Model file for the job. Use its own axes, mm. A direction names the side the tool comes from. Coordinates: 2 decimals unless noted, no trailing zeros. Order: outer loops, then holes, each group sorted by start corner. A loop starts at its lowest first (then second) coordinate and runs counter-clockwise, first axis right, second up. Notation, with made-up numbers: (-33.5, -25.75) -> (-0.5, -25.75) arc R32 ccw to (-0.5, 11.25) -> close; hole circle Ø11 at (4, -0.5). An arc over 180 degrees is marked (long way). Return JSON: item names as keys, results as strings. Group by question number.
1) Cut at B-B (x = -70). Write the cut outline in (y, z), and give its area (3 significant figures).
2) Cut at C-C (z = 0). State how many separate pieces and enclosed holes the cut face has, and give its area (3 significant figures).
3) Pull direction Z, two halves, no side cores. Call faces 1 (the flat face through (-20.5, -38, 0)), 2 (the cylindrical face through (59, 13, 0)): +Z half, -Z half, draft (parallel to the pull), parting line (faces both ways), or undercut.
4) Flat gauge pins, fed straight in: pin 1 (16 mm diameter, centred on y = 52.5, z = 3, fed in from +X); pin 2 (12 mm diameter, centred on y = -60.5, z = 2, fed in from -X); pin 3 (12 mm diameter, centred on x = -80, z = -4, fed in from +Y). Where does each tip first touch, or does it go through?
5) Which spindle directions (+Z, -Z, +X, -X, +Y, -Y) get a long thin tool onto all of the face, cutting with end or side? Do faces 3 (the flat face through (61, -20, 9)), 4 (the flat face through (-80, 20, 9)), 5 (the flat face through (25, 75, 0)), 6 (the flat face through (85.5, 0, 0)), 7 (the flat face through (-20.5, 53, 0)). Say none if no direction does.
6) Probe line 1 (X direction, y = 14.5, z = 0); line 2 (X direction, y = -15.75, z = 0); line 3 (Z direction, x = 70, y = -10.25). List the from-to ranges inside material, lowest first.
7) Cut at A-A (y = -47). Write the cut outline in (x, z).
from build123d import *

# Parameters (mm, degrees)
F0_W      = 60
F0_H      = 40
F1_DEPTH  = 90
F2_W      = 41
F2_H      = 40
F3_DEPTH  = 80
F4_W      = 41
F4_H      = 40
F5_DEPTH  = 80
F6_W      = 75
F6_H      = 40
F6_R      = 11
F7_DEPTH  = 20
F8_W      = 31
F8_H      = 12
F9_DEPTH  = 40
F10_R     = 20
F11_R     = 5
F12_R     = 5
F13_W     = 5
F13_H     = 30
F14_DEPTH = 80


with BuildPart() as f1:
    # F0 (on Front) → F1 (new body, symmetric)
    with BuildSketch(Plane.XZ):
        Rectangle(F0_W, F0_H)
    extrude(amount=F1_DEPTH, both=True)

    # F2 (on face) → F3 (cut)
    with BuildSketch(Plane.XZ.offset(90)):
        Rectangle(F2_W, F2_H)
    extrude(amount=-F3_DEPTH, mode=Mode.SUBTRACT)

    # F4 (on face) → F5 (cut)
    with BuildSketch(Plane(origin=(0, 90, 0), x_dir=(-1, 0, 0), z_dir=(0, 1, 0))):
        Rectangle(F4_W, F4_H)
    extrude(amount=-F5_DEPTH, mode=Mode.SUBTRACT)

    # F6 (on Front) → F7 (join, symmetric)
    with BuildSketch(Plane.XZ):
        with Locations((58, 0)):
            Rectangle(F6_W, F6_H)
        with Locations((70, 0)):
            Circle(F6_R, mode=Mode.SUBTRACT)
        with Locations((-58, 0)):
            Rectangle(F6_W, F6_H)
        with Locations((-70, 0)):
            Circle(F6_R, mode=Mode.SUBTRACT)
    extrude(amount=F7_DEPTH, both=True)

    # F8 (on face) → F9 (cut)
    with BuildSketch(Plane.XY.offset(20)):
        with Locations((70, 0)):
            Rectangle(F8_W, F8_H)
        with Locations((-70, 0)):
            Rectangle(F8_W, F8_H)
    extrude(amount=-F9_DEPTH, mode=Mode.SUBTRACT)

    # F10
    f10_edges = [f1.edges().sort_by_distance(p)[0] for p in [
        (-30, -20, 0),
        (30, -20, 0),
        (-30, 20, 0),
        (30, 20, 0),
    ]]
    fillet(f10_edges, radius=F10_R)

    # F11
    f11_edges = [f1.edges().sort_by_distance(p)[0] for p in [
        (-95.5, 20, 0),
        (-95.5, -20, 0),
        (95.5, -20, 0),
        (95.5, 20, 0),
    ]]
    fillet(f11_edges, radius=F11_R)

    # F12
    f12_edges = [f1.edges().sort_by_distance(p)[0] for p in [
        (-20.5, -10, 0),
        (-20.5, 10, 0),
        (20.5, 10, 0),
        (20.5, -10, 0),
    ]]
    fillet(f12_edges, radius=F12_R)

    # F13 (on face) → F14 (cut)
    with BuildSketch(Plane.XY.offset(20)):
        with Locations((-27.5, 75)):
            Rectangle(F13_W, F13_H)
        with Locations((27.5, 75)):
            Rectangle(F13_W, F13_H)
        with Locations((-23, -75)):
            Rectangle(F13_W, F13_H)
        with Locations((23, -75)):
            Rectangle(F13_W, F13_H)
    extrude(amount=-F14_DEPTH, mode=Mode.SUBTRACT)


solid = f1.part
Answers below:
{
 "1": {"outline": "(-20, -20) -> (-6, -20) -> (-6, -11) -> (-20, -11) -> close; (-20, 11) -> (-6, 11) -> (-6, 20) -> (-20, 20) -> close; (6, -20) -> (20, -20) -> (20, -11) -> (6, -11) -> close; (6, 11) -> (20, 11) -> (20, 20) -> (6, 20) -> close", "area": "504 mm^2"},
 "2": {"separate pieces": "3", "enclosed holes": "0", "area": "7,250 mm^2"},
 "3": {"face 1": "draft", "face 2": "undercut"},
 "4": {"pin 1": "stops at x = 30", "pin 2": "stops at x = -30", "pin 3": "stops at y = 20"},
 "5": {"face 3": "+Z, -Z, +X, -Y", "face 4": "+Z, -Z, -X, +Y", "face 5": "+Z, -Z, +X, +Y", "face 6": "+Z, -Z", "face 7": "+Z, -Z, +Y"},
 "6": {"line 1": "x = -95.5 to -81, -59 to -20.47, 20.47 to 59, 81 to 95.5", "line 2": "x = -95.44 to -81, -59 to -20.5, 20.5 to 59, 81 to 95.44", "line 3": "z = -20 to -11, 11 to 20"},
 "7": {"outline": "(-30, -20) -> (-20.5, -20) -> (-20.5, 20) -> (-30, 20) -> close; (20.5, -20) -> (30, -20) -> (30, 20) -> (20.5, 20) -> close"}
}
